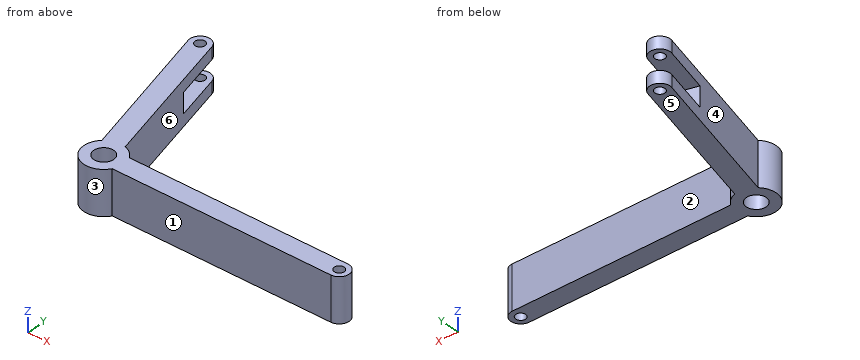
```python
from build123d import *

# Parameters (mm, degrees)
SKETCH_1_R          = 2.5
SKETCH_1_R_2        = 5
EXTRUDE_1_DEPTH     = 11
SKETCH_1_2_R        = 5
SKETCH_1_2_R_2      = 2.5
EXTRUDE_2_DEPTH     = 11
SKETCH_3_R          = 2.5
CUT_EXTRUDE_1_DEPTH = 5


with BuildPart() as part:
    # 草图1 → 凸台-拉伸1 (new, symmetric)
    with BuildSketch(Plane.XY):
        with BuildLine():
            Line((82.916122479, 118.415426808), (102.598160303, 44.656581333))
            ThreePointArc((102.598160303, 44.656581333), (106.091708364, 42.93039023), (108.660254038, 40))
            Line((108.660254038, 40), (220, 40))
            ThreePointArc((220, 40), (225, 35), (220, 30))
            Line((220, 30), (108.660254038, 30))
            ThreePointArc((108.660254038, 30), (93.916481406, 27.063325538), (92.921636508, 42.063764596))
            Line((92.921636508, 42.063764596), (73.087358524, 115.781817444))
            ThreePointArc((73.087358524, 115.781817444), (76.683575783, 122.01807983), (82.916122479, 118.415426808))
        make_face()
        with Locations((78.000381166, 117.103695235)):
            Circle(SKETCH_1_R, mode=Mode.SUBTRACT)
        with Locations((220, 35)):
            Circle(SKETCH_1_R, mode=Mode.SUBTRACT)
        with Locations((100, 35)):
            Circle(SKETCH_1_R_2, mode=Mode.SUBTRACT)
    extrude(amount=EXTRUDE_1_DEPTH, both=True)

    # 草图1<2> → 凸台-拉伸2 (add, symmetric)
    with BuildSketch(Plane.XY):
        with BuildLine():
            Line((102.598160303, 44.656581333), (82.916122479, 118.415426808))
            ThreePointArc((82.916122479, 118.415426808), (76.683575783, 122.01807983), (73.087358524, 115.781817444))
            Line((73.087358524, 115.781817444), (92.921636508, 42.063764596))
            ThreePointArc((92.921636508, 42.063764596), (93.916481406, 27.063325538), (108.660254038, 30))
            Line((108.660254038, 30), (220, 30))
            ThreePointArc((220, 30), (225, 35), (220, 40))
            Line((220, 40), (108.660254038, 40))
            ThreePointArc((108.660254038, 40), (106.091708364, 42.93039023), (102.598160303, 44.656581333))
        make_face()
        with Locations((100, 35)):
            Circle(SKETCH_1_2_R, mode=Mode.SUBTRACT)
        with Locations((220, 35)):
            Circle(SKETCH_1_2_R_2, mode=Mode.SUBTRACT)
        with Locations((78.000381166, 117.103695235)):
            Circle(SKETCH_1_2_R_2, mode=Mode.SUBTRACT)
    extrude(amount=EXTRUDE_2_DEPTH, both=True)

    # 草图3 → 切除-拉伸1 (cut, symmetric)
    with BuildSketch(Plane.XY):
        with BuildLine():
            Line((89.361667081, 94.260614559), (82.916122479, 118.415426808))
            ThreePointArc((82.916122479, 118.415426808), (76.683575783, 122.01807983), (73.087358524, 115.781817444))
            Line((73.087358524, 115.781817444), (79.580043978, 91.650456081))
            Line((79.580043978, 91.650456081), (89.361667081, 94.260614559))
        make_face()
        with Locations((78.000381166, 117.103695235)):
            Circle(SKETCH_3_R, mode=Mode.SUBTRACT)
    extrude(amount=CUT_EXTRUDE_1_DEPTH, both=True, mode=Mode.SUBTRACT)


solid = part.part
```
The model under review builds one solid part; all positions refer to its coordinate system, in mm. Face numbers are marked on the shaded views. A direction names the side the tool comes from. Round coordinates to 2 decimals unless told otherwise and drop trailing zeros. Write each loop counter-clockwise with the first axis right and the second up, starting at its lowest first coordinate (ties: lowest second). Pieces come first, ordered by that corner, then holes. Notation, with made-up numbers: (63, 86) - (87, 86) arc R21 cw to (87, 101) - close; hole circle Ø6 at (11.25, -21.75). An arc over 180 degrees is marked (long way). Answer as CSV lines item,"result". Start each with the question number.
(1) We need section C-C on x = 100. State the section outline as (y, z) points, plus the area to 3 significant figures.
(2) We need section B-B on z = 1.75. State the section outline as (x, y) points.
(3) To check wall thickness, follow line 1 (Y direction, x = 220, z = 6.5); line 2 (Y direction, x = 141.5, z = -4.25); line 3 (X direction, y = 118, z = -6.5). State the ranges of each line that lie inside material, in increasing order.
(4) For the marked faces 1, 2 and 3, list the 3-axis set-ups (+Z, -Z, +X, -X, +Y, -Y) from which the entire face can be reached by the end or side of a thin tool; tool diameter is ignored.
(5) Draft analysis for pull direction Y (two halves, no side actions). For the marked faces 4, 5 and 6, state which applies: pulls with the +Y half, pulls with the -Y half, needs draft (parallel to the pull), parting line crosses it, or undercut.
(6) We need section D-D on y = 103. State the section outline as (x, z) points, plus the area to 3 significant figures.
(7) For pin 1 Ø4 at (y, z) = (57.5, 7) entering from -X; pin 2 Ø6.5 at (x, z) = (154.5, -2.5) entering from -Y; pin 3 Ø10 at (x, z) = (108.5, 3.5) entering from -Y; pin 4 Ø4.5 at (x, y) = (78, 117.1) entering from -Z, all flat-tipped, find the tip position at first contact; note any pin that passes through.
(8) We need section A-A on y = 35. State the section outline as (x, z) points, plus the area to 3 significant figures.
Worked answers:
1,outline,"(25, -11) - (30, -11) - (30, 11) - (25, 11) - close; (40, -11) - (54.39, -11) - (54.39, 11) - (40, 11) - close"
1,area,"427 mm²"
2,outline,"(79.58, 91.65) - (92.92, 42.06) arc R10 ccw (long way) to (108.66, 30) - (220, 30) arc R5 ccw to (220, 40) - (108.66, 40) arc R10 ccw to (102.6, 44.66) - (89.36, 94.26) - close; hole circle Ø10 at (100, 35); hole circle Ø5 at (220, 35)"
3,line 1,"30 to 32.5, 37.5 to 40"
3,line 2,"30 to 40"
3,line 3,"72.99 to 75.67, 80.33 to 83.03"
4,face 1,"+Z, -Z, +X, -Y"
4,face 2,"+Z, -Z, +X, +Y"
4,face 3,"+Z, -Z"
5,face 4,"undercut"
5,face 5,"needs draft"
5,face 6,"pulls with the +Y half"
6,outline,"(76.53, -11) - (87.03, -11) - (87.03, -5) - (76.53, -5) - close; (76.53, 5) - (87.03, 5) - (87.03, 11) - (76.53, 11) - close"
6,area,"126 mm²"
7,pin 1,"x = 88.23"
7,pin 2,"y = 30"
7,pin 3,"y = 25.63"
7,pin 4,"through"
8,outline,"(90, -11) - (95, -11) - (95, 11) - (90, 11) - close; (105, -11) - (217.5, -11) - (217.5, 11) - (105, 11) - close; (222.5, -11) - (225, -11) - (225, 11) - (222.5, 11) - close"
8,area,"2,640 mm²"
